Build history of the part. All positions in model axes, mm. A direction names the side the tool comes from. Round coordinates to 2 decimals unless told otherwise and drop trailing zeros. Write each loop counter-clockwise with the first axis right and the second up, starting at its lowest first coordinate (ties: lowest second). Pieces come first, ordered by that corner, then holes. Notation, with made-up numbers: M -20,59 L -15,59 A23 cw -15,84 Z; hole C -24,7.25 d5. An arc over 180 degrees is marked long. Use a Markdown table: item, result.
from build123d import *

# Parameters (mm, degrees)
PAD004_DEPTH      = 0.6
PAD004_DEPTH_BACK = 7
FILLET001_R       = 1
FILLET002_R       = 0.5
THICKNESS002_T    = -0.3


with BuildPart() as part:
    # Sketch006 (on Face1 of ReferenceLinearPattern004) → Pad004 (new body, two sides)
    with BuildSketch(Plane.XZ) as pad004_sk:
        Polygon((18, 4.5), (6.8, 4.5), (6.8, 2.2), (8.8, 1), (16, 1), (18, 2.2), align=None)
    extrude(amount=PAD004_DEPTH)
    extrude(pad004_sk.sketch, amount=-PAD004_DEPTH_BACK)

    # Fillet001
    fillet001_edges = [part.edges().sort_by_distance(p)[0] for p in [
        (6.8, 3.2, 4.5),
        (18, 3.2, 4.5),
    ]]
    fillet(fillet001_edges, radius=FILLET001_R)

    # Fillet002
    fillet002_edges = [part.edges().sort_by_distance(p)[0] for p in [
        (6.8, 3.2, 2.2),
        (8.8, 3.2, 1),
        (16, 3.2, 1),
        (18, 3.2, 2.2),
    ]]
    fillet(fillet002_edges, radius=FILLET002_R)

    # Thickness002
    thickness002_openings = [part.faces().sort_by_distance(p)[0] for p in [
        (12.4, -0.6, 2.821651),
    ]]
    offset(amount=THICKNESS002_T, openings=thickness002_openings)


solid = part.part
Q1. Two-plate mould, pull along X, no slides. Class faces 1 (the flat face through (12, 3, 1.3)), 2 (the flat face through (12, 7, 3)), 3 (the cylindrical face through (7.101, 3.147, 4.215)), 4 (the flat face through (7.1, 3, 3)): +X half, -X half, draft (parallel to the pull), parting line (faces both ways), or undercut.
Response values:
| item | result |
|---|---|
| face 1 | undercut |
| face 2 | draft |
| face 3 | -X half |
| face 4 | undercut |
Q2. Cut at A-A on y = 3.75. Give the cut face in (x, z).
Response values:
| item | result |
|---|---|
| outline | M 6.8,2.48 A0.5 ccw 7.04,2.05 L 8.68,1.07 A0.5 ccw 8.94,1 L 15.86,1 A0.5 ccw 16.12,1.07 L 17.76,2.05 A0.5 ccw 18,2.48 L 18,3.5 A1 ccw 17,4.5 L 7.8,4.5 A1 ccw 6.8,3.5 Z; hole M 7.1,2.48 A0.2 ccw 7.2,2.31 L 8.84,1.33 A0.2 ccw 8.94,1.3 L 15.86,1.3 A0.2 ccw 15.96,1.33 L 17.6,2.31 A0.2 ccw 17.7,2.48 L 17.7,3.5 A0.7 ccw 17,4.2 L 7.8,4.2 A0.7 ccw 7.1,3.5 Z |
Q3. Which spindle directions (+Z, -Z, +X, -X, +Y, -Y) get a long thin tool onto all of the face, cutting with end or side? Do faces 5 (the flat face through (17.7, 3, 3)), 6 (the flat face through (12, 3, 1)). Say none if no direction does.
Response values:
| item | result |
|---|---|
| face 5 | -Y |
| face 6 | -Z, +X, -X, +Y, -Y |
Q4. Drop a flat-ended pin along its axis: P1, Ø1, axis at y = 5, z = 4, coming from the -X side. Give the stop position or say it passes through.
Response values:
| item | result |
|---|---|
| P1 | stops at x = 6.8 |
Q5. Cut at B-B on x = 13.5. Give the cut face in (y, z), and give its area (3 significant figures).
Response values:
| item | result |
|---|---|
| outline | M -0.6,1 L 7,1 L 7,4.5 L -0.6,4.5 L -0.6,4.2 L 6.7,4.2 L 6.7,1.3 L -0.6,1.3 Z |
| area | 5.43 mm2 |
Q6. Drill centre lines: L1, parallel to Z at x = 10.25, y = 0; L2, parallel to X at y = 2.75, z = 3.55; L3, parallel to Y at x = 8.5, z = 2.2. Where is each one in solid material? Low to high.
Response values:
| item | result |
|---|---|
| L1 | z = 1 to 1.3, 4.2 to 4.5 |
| L2 | x = 6.8 to 7.1, 17.7 to 18 |
| L3 | y = 6.7 to 7 |
Q7. Cut at C-C on z = 3.3. Give the cut face in (x, y).
Response values:
| item | result |
|---|---|
| outline | M 6.8,-0.6 L 7.1,-0.6 L 7.1,6.7 L 17.7,6.7 L 17.7,-0.6 L 18,-0.6 L 18,7 L 6.8,7 Z |
